Autodesk Inventor part; units mm, degrees
ref_plane "YZ Plane" through (0, 0, 0) normal (1, 0, 0) x (0, 1, 0)
ref_plane "XZ Plane" through (0, 0, 0) normal (0, 1, 0) x (-1, 0, 0)
ref_plane "XY Plane" through (0, 0, 0) normal (0, 0, 1) x (1, 0, 0)
sketch "Sketch1" plane through (0, 0, 0) normal (0, 1, 0) x (-1, 0, 0)
  arc A0 (3.8932, 5.0165) -> (4.9314, -4.0005) centre (0, 0) ccw
  arc A1 (3.2922, 0.254) -> (3.2627, -0.508) centre (0, 0) ccw
  line L0 (14.605, -0.508) -> (14.605, -4.0005)
  line L1 (14.605, -4.0005) -> (4.9314, -4.0005)
  line L2 (14.605, 0.254) -> (14.605, 5.0165)
  line L3 (14.605, 5.0165) -> (3.8932, 5.0165)
  line L4 (3.2627, -0.508) -> (14.605, -0.508)
  line L5 (3.2922, 0.254) -> (14.605, 0.254)
  dimension "d0" = 12.7
  dimension "d1" = 6.604
  dimension "d8" = 0.254
  dimension "d9" = 0.508
  dimension "d10" = 4.7625
  dimension "d11" = 3.4925
  dimension "d25" = 14.605
  dimension "d26" = 14.605
extrude "PartShape" add sketch "Sketch1" along normal blind 7.62
sketch "Sketch2" plane through (0, 7.62, 0) normal (0, 1, 0) x (1, 0, 0)
  arc A0 (-3.9288, -0.254) -> (-3.9041, 0.508) centre (0, 0) ccw
  arc A1 (-3.2922, -0.254) -> (-3.2627, 0.508) centre (0, 0) ccw
  line L0 (-3.2922, -0.254) -> (-14.605, -0.254)
  line L1 (-3.9288, -0.254) -> (-3.2922, -0.254)
  line L2 (-14.605, 0.508) -> (-3.2627, 0.508)
  arc A2 (-3.2922, -0.254) -> (-3.2627, 0.508) centre (0, 0) ccw
  line L3 (-14.605, 0.508) -> (-3.2627, 0.508)
  line L4 (-3.9041, 0.508) -> (-3.2627, 0.508)
  dimension "d14" = 7.874
extrude "RaceStandoff" add sketch "Sketch2" along normal blind 0.762
sketch "Sketch3" plane through (-14.605, 0, 5.0165) normal (0, 0, 1) x (1, 0, 0)
  line L0 (0, 0) -> (0, 7.62) construction
  line L1 (0, 3.81) -> (11.9818, 3.81) construction
  line L2 (10.7118, 0) -> (10.7118, 7.62) construction
  circle A0 centre (6.0509, 3.81) radius 4.6609 construction
  line L3 (6.0509, -0.8509) -> (2.0144, 1.4796)
  line L4 (2.0144, 1.4796) -> (2.0144, 6.1404)
  line L5 (2.0144, 6.1404) -> (6.0509, 8.4709)
  line L6 (6.0509, 8.4709) -> (10.0873, 6.1405)
  line L7 (10.0873, 6.1405) -> (10.0873, 1.4796)
  line L8 (10.0873, 1.4796) -> (6.0509, -0.8509)
  point P0 (14.605, 0)
  dimension "d18" = 9.3218
  dimension "d19" = 4.6609
extrude "NutWell" cut sketch "Sketch3" against normal blind 3.81
sketch "Sketch4" plane through (-14.605, 0, 1.2065) normal (0, 0, 1) x (1, 0, 0)
  line L0 (10.7118, 0) -> (10.7118, 7.62) construction
  line L1 (10.6762, 7.62) -> (0, 7.62) construction
  circle A0 centre (6.0509, 3.81) radius 1.9304
  line L2 (2.0144, 6.1404) -> (4.5771, 7.62) construction
  line L3 (10.0873, 6.1405) -> (10.0873, 1.4796) construction
  line L4 (2.0144, 6.1404) -> (10.0873, 1.4796) construction
  line L5 (10.0873, 1.4796) -> (10.0873, 6.1404) construction
  line L6 (4.5771, 0) -> (2.0144, 1.4796) construction
  line L7 (10.0873, 6.1404) -> (2.0144, 1.4796) construction
  point P0 (14.605, 0)
  point P1 (11.9818, 3.81)
  point P2 (12.5191, 7.62)
  dimension "d22" = 3.8608
extrude "ScrewHole" cut sketch "Sketch4" against normal through all
fillet "Fillet1" radius 1.27 1 edges at (-4.9314, 3.81, -4.0005)
fillet "Fillet2" radius 1.778 1 edges at (-3.8932, 3.81, 5.0165)
properties part number "Clamping Collar 1_4"
Could you check a few things on this model? Use its own coordinates, in mm. A direction names the side the tool comes from. Give positions to 0.01 mm unless a question says otherwise; leave off trailing zeros. Order: outer loops, then holes, each group sorted by start corner. A loop starts at its lowest first (then second) coordinate and runs counter-clockwise, first axis right, second up.
Q1. Suppose I cut it at A-A, the plane y = 3.81. Count the separate pieces of the cut face and the enclosed holes in it, and give its area (3 significant figures).
Q2. Suppose I cut it at D-D, the plane x = -1.25. Write out the boundary of the cut face in (y, z).
Q3. I'm going to push flat-ended pins straight in: P1, Ø4, axis at x = -9, y = 4, coming from the +Z side; P2, Ø4, axis at y = 7.5, z = 2.5, coming from the +X side; P3, Ø3, axis at y = 3, z = 3.5, coming from the +X side. Where does each tip first touch, or does it pass through?
Q4. Suppose I cut it at C-C, the plane x = -8.75. Write out the boundary of the cut face in (y, z).
Q5. We'd pull the mould along Y, two halves only. Please class faces 1 (the flat face through (-14.605, 4, -2)), 2 (the flat face through (-8, 6, 1.206)), 3 (the flat face through (-2, 8.382, 3)), 4 (the flat face through (-11.29, 0.73, 3.14)): +Y half, -Y half, draft (parallel to the pull), parting line (faces both ways), or undercut.
Q6. Suppose I cut it at B-B, the plane z = -1.5. Write out the boundary of the cut face in (x, y) (3 decimals).
Q7. For faces 5 (the flat face through (-10, 2, -0.508)), 6 (the flat face through (-4, 7.62, 1)), 7 (the flat face through (-13, 4, 5.016)), 8 (the flat face through (-11.33, 6.87, 3.14)), 9 (the flat face through (-11, 4, -4)), which set-ups out of +Z, -Z, +X, -X, +Y, -Y let a thin tool reach every point of the face, with its end or its side?
Q8. If I drill on line 1 along Z through (x, y) = (-11, 1.5); line 2 along X through (y, z) = (6.25, 3) (3 decimals); line 3 along X through (y, z) = (5.5, -2.5) (3 decimals), over which ranges is the centre line in solid material (lowest first)?
Solution:
1. separate pieces: 3
1. enclosed holes: 0
1. area: 116 mm2
2. outline: (0, -6.23) - (7.62, -6.23) - (7.62, -3.73) - (8.38, -3.73) - (8.38, -3.06) - (0, -3.06) - close; (0, 3.06) - (8.38, 3.06) - (8.38, 3.73) - (7.62, 3.73) - (7.62, 6.23) - (0, 6.23) - close
3. P1: stops at z = 1.21
3. P2: stops at x = 6.33
3. P3: stops at x = 6.03
4. outline: (0, -4) - (1.89, -4) - (1.89, -0.51) - (0, -0.51) - close; (0, 0.25) - (1.89, 0.25) - (1.89, 1.21) - (0, 1.21) - close; (5.73, -4) - (7.62, -4) - (7.62, -0.51) - (5.73, -0.51) - close; (5.73, 0.25) - (7.62, 0.25) - (7.62, 1.21) - (5.73, 1.21) - close
5. face 1: draft
5. face 2: undercut
5. face 3: +Y half
5. face 4: undercut
6. outline: (-14.605, 0) - (-2.942, 0) - (-2.942, 8.382) - (-3.64, 8.382) - (-3.64, 7.62) - (-14.605, 7.62) - close; (2.942, 0) - (6.17, 0) - (6.17, 7.62) - (3.64, 7.62) - (3.64, 8.382) - (2.942, 8.382) - close; hole circle Ø3.861 at (-8.554, 3.81)
7. face 5: -X, +Y, -Y
7. face 6: +Y
7. face 7: +Z, -X, +Y, -Y
7. face 8: +Z
7. face 9: -Z, -X, +Y, -Y
8. line 1: z = -4 to -0.51, 0.25 to 1.21
8. line 2: x = -14.605 to -12.401, -4.707 to -1.379, 1.379 to 5.597
8. line 3: x = -14.605 to -9.487, -7.621 to -2.157, 2.157 to 5.837
